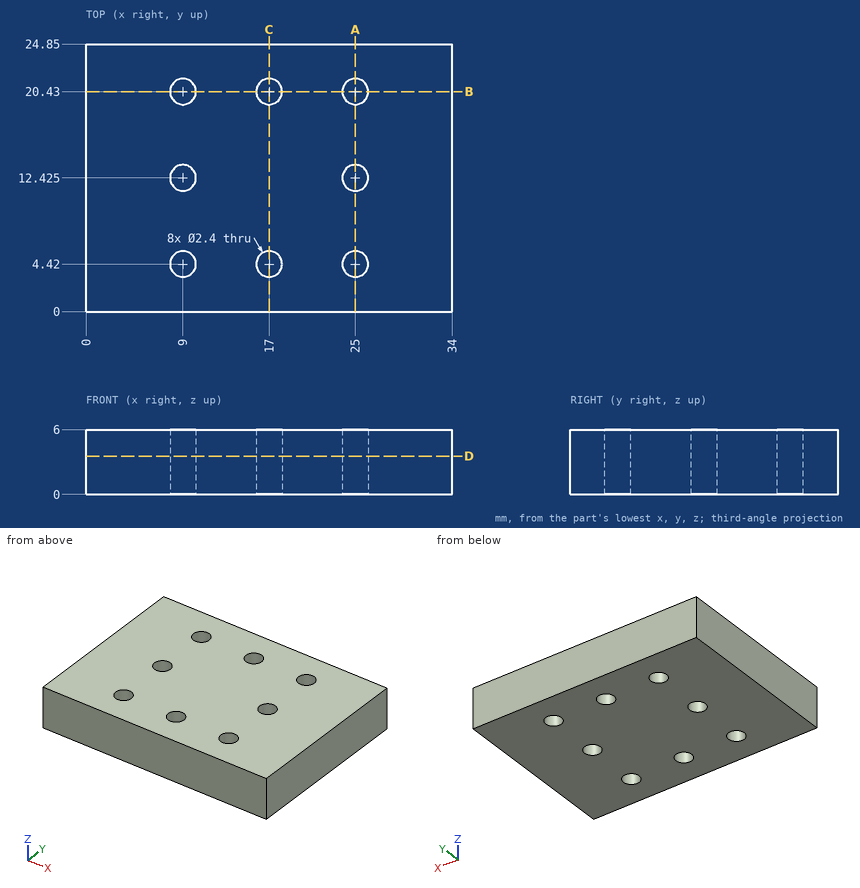
Design review of the part shown in the three views and the two pictorial views. Dimensions are in mm from the part's minimum x, y and z. Round coordinates to 2 decimals unless told otherwise and drop trailing zeros. Order: outer loops, then holes, each group sorted by start corner. A loop starts at its lowest first (then second) coordinate and runs counter-clockwise, first axis right, second up. Notation, with made-up numbers: M -11,56.25 L 4,56.25 A8 cw 4,61.25 Z; hole C 2,64.5 d3. An arc over 180 degrees is marked long. Put each result on its own line as item: value.
Q1. Consider section D-D (z = 3.55). State how many separate pieces and enclosed holes the cut face has, and give its area (3 significant figures).
Reported:
separate pieces: 1
enclosed holes: 8
area: 809 mm²
Q2. Consider section C-C (x = 17). State the section outline as (y, z) points, and give its area (3 significant figures).
Reported:
outline: M 0,0 L 3.22,0 L 3.22,6 L 0,6 Z; M 5.62,0 L 19.23,0 L 19.23,6 L 5.62,6 Z; M 21.63,0 L 24.85,0 L 24.85,6 L 21.63,6 Z
area: 120 mm²
Q3. Insertion check: pin 1 Ø1.4 at (x, y) = (25, 4.42) entering from -Z. The pin has a flat end and moves straight along its axis. Give the tip position at first contact, or say it passes through.
Reported:
pin 1: through
Q4. Consider section B-B (y = 20.43). State the section outline as (x, z) points.
Reported:
outline: M 0,0 L 7.8,0 L 7.8,6 L 0,6 Z; M 10.2,0 L 15.8,0 L 15.8,6 L 10.2,6 Z; M 18.2,0 L 23.8,0 L 23.8,6 L 18.2,6 Z; M 26.2,0 L 34,0 L 34,6 L 26.2,6 Z
Q5. To check wall thickness, follow line 1 (Y direction, x = 17, z = 3.25); line 2 (Y direction, x = 25, z = 3.1) (3 decimals); line 3 (X direction, y = 12.25, z = 0.4). State the ranges of each line that lie inside material, in increasing order.
Reported:
line 1: 0 to 3.22, 5.62 to 19.23, 21.63 to 24.85
line 2: 0 to 3.22, 5.62 to 11.225, 13.625 to 19.23, 21.63 to 24.85
line 3: 0 to 7.81, 10.19 to 23.81, 26.19 to 34
Q6. Consider section A-A (x = 25). State the section outline as (y, z) points (3 decimals).
Reported:
outline: M 0,0 L 3.22,0 L 3.22,6 L 0,6 Z; M 5.62,0 L 11.225,0 L 11.225,6 L 5.62,6 Z; M 13.625,0 L 19.23,0 L 19.23,6 L 13.625,6 Z; M 21.63,0 L 24.85,0 L 24.85,6 L 21.63,6 Z
